```python
from build123d import *

# Parameters (mm, degrees)
SKETCH1_R                                    = 18.5
SKETCH1_R_2                                  = 2.125
MAIN_DEPTH                                   = 2
INLET_FILLET_R                               = 5
SKETCH20_R                                   = 8.5
FAN_PROTECTION_RIBS_DEPTH                    = 2
FAN_PROTECTION_RIBS_FILLETS_R                = 2
CSK_FOR_M4_HEX_SOCKET_COUNTERSUNK_HE_2_COUNT = 2
CSK_FOR_M4_HEX_SOCKET_COUNTERSUNK_HE_2_PITCH = 79.5
CSK_FOR_M4_HEX_SOCKET_COUNTERSUNK_HE_3_COUNT = 2
CSK_FOR_M4_HEX_SOCKET_COUNTERSUNK_HE_3_PITCH = 105.5
CSK_FOR_M4_HEX_SOCKET_COUNTERSUNK_HE_4_COUNT = 2
CSK_FOR_M4_HEX_SOCKET_COUNTERSUNK_HE_4_PITCH = 132.10034065


with BuildPart() as part:
    # Sketch1 → Main (new body)
    with BuildSketch(Plane.XY):
        with BuildLine():
            Line((-42.95, -46.393826455), (62.55, -46.393826455))
            ThreePointArc((62.55, -46.393826455), (67.782590181, -44.226416636), (69.95, -38.993826455))
            Line((69.95, -38.993826455), (69.95, 40.506173545))
            ThreePointArc((69.95, 40.506173545), (67.782590181, 45.738763726), (62.55, 47.906173545))
            Line((62.55, 47.906173545), (11.070508076, 47.906173545))
            Line((11.070508076, 47.906173545), (-23.570508076, 47.906173545))
            Line((-23.570508076, 47.906173545), (-42.95, 47.906173545))
            ThreePointArc((-42.95, 47.906173545), (-48.182590181, 45.738763726), (-50.35, 40.506173545))
            Line((-50.35, 40.506173545), (-50.35, -38.993826455))
            ThreePointArc((-50.35, -38.993826455), (-48.182590181, -44.226416636), (-42.95, -46.393826455))
        make_face()
        with Locations((-4.75, 17)):
            Circle(SKETCH1_R, mode=Mode.SUBTRACT)
        with Locations((-42.95, 40.506173545)):
            Circle(SKETCH1_R_2, mode=Mode.SUBTRACT)
        with Locations((-42.95, -38.993826455)):
            Circle(SKETCH1_R_2, mode=Mode.SUBTRACT)
        with Locations((62.55, 40.506173545)):
            Circle(SKETCH1_R_2, mode=Mode.SUBTRACT)
        with Locations((62.55, -38.993826455)):
            Circle(SKETCH1_R_2, mode=Mode.SUBTRACT)
    extrude(amount=-MAIN_DEPTH)

    # Inlet Fillet
    # the kernel refuses this fillet: 5 mm, written as the material it takes off along each edge
    with BuildSketch(Plane(origin=(-4.75, 17, 0), x_dir=(1, 0, 0), z_dir=(0, -1, 0))) as inlet_fillet_piece_1:
        with BuildLine():
            CenterArc((22.5, -5), INLET_FILLET_R, 90, 53.130102354)
            Line((22.5, 0), (22.5, 0.1))
            Line((22.5, 0.1), (18.5, 0.1))
            Line((18.5, 0.1), (18.4, 0))
            ThreePointArc((18.4, 0), (18.4, -1), (18.42, -1.94))
            Line((18.42, -1.94), (18.5, -2))
        make_face()
    revolve(axis=Axis((-4.75, 17, 0), (0, 0, 1)), mode=Mode.SUBTRACT)

    # Sketch20 → Fan Protection Ribs (add, through all)
    with BuildSketch(Plane.XY):
        with Locations((-4.75, 17)):
            Circle(SKETCH20_R)
        with BuildLine():
            ThreePointArc((-5.35, 25.478797084), (-4.75, 25.5), (-4.15, 25.478797084))
            Line((-4.15, 25.478797084), (-4.15, 39.491998577))
            ThreePointArc((-4.15, 39.491998577), (-4.75, 39.5), (-5.35, 39.491998577))
            Line((-5.35, 39.491998577), (-5.35, 25.478797084))
        make_face()
        with BuildLine():
            Line((15.02864215, 6.273615954), (2.892853669, 13.2802167))
            ThreePointArc((2.892853669, 13.2802167), (2.611215932, 12.75), (2.292853669, 12.240986215))
            Line((2.292853669, 12.240986215), (14.42864215, 5.234385469))
            ThreePointArc((14.42864215, 5.234385469), (14.735571585, 5.75), (15.02864215, 6.273615954))
        make_face()
        with BuildLine():
            ThreePointArc((-11.792853669, 12.240986215), (-12.111215932, 12.75), (-12.392853669, 13.2802167))
            Line((-12.392853669, 13.2802167), (-24.52864215, 6.273615954))
            ThreePointArc((-24.52864215, 6.273615954), (-24.235571585, 5.75), (-23.92864215, 5.234385469))
            Line((-23.92864215, 5.234385469), (-11.792853669, 12.240986215))
        make_face()
    extrude(amount=-FAN_PROTECTION_RIBS_DEPTH)

    # Fan Protection Ribs Fillets
    fan_protection_ribs_fillets_edges = [part.edges().sort_by_distance(p)[0] for p in [
        (-4.15, 25.478797084, -1),
        (2.892853669, 13.2802167, -1),
        (2.292853669, 12.240986215, -1),
        (-11.792853669, 12.240986215, -1),
        (-12.392853669, 13.2802167, -1),
        (-5.35, 25.478797084, -1),
    ]]
    fillet(fan_protection_ribs_fillets_edges, radius=FAN_PROTECTION_RIBS_FILLETS_R)

    # Sketch23 → CSK for M4 Hex Socket Countersunk Head Screw3 (revolve, cut)
    with BuildSketch(Plane(origin=(-42.95, 40.506173545, 0), x_dir=(0, -1, 0), z_dir=(1, 0, 0))):
        Polygon((0, 0), (0, 2), (2.15, 2), (2.15, 2.44), (4.59, 0), align=None)
    csk_for_m4_hex_socket_countersunk_head_s = revolve(axis=Axis((-42.95, 40.506173545, 6.35), (0, 0, -1)), mode=Mode.SUBTRACT)

    # CSK for M4 Hex Socket Countersunk He 2: CSK for M4 Hex Socket Countersunk Head Screw3 ×2
    with Locations(*[(0, -i * CSK_FOR_M4_HEX_SOCKET_COUNTERSUNK_HE_2_PITCH, 0) for i in range(1, CSK_FOR_M4_HEX_SOCKET_COUNTERSUNK_HE_2_COUNT)]):
        add(csk_for_m4_hex_socket_countersunk_head_s, mode=Mode.SUBTRACT)

    # CSK for M4 Hex Socket Countersunk He 3: CSK for M4 Hex Socket Countersunk Head Screw3 ×2
    with Locations(*[(i * CSK_FOR_M4_HEX_SOCKET_COUNTERSUNK_HE_3_PITCH, 0, 0) for i in range(1, CSK_FOR_M4_HEX_SOCKET_COUNTERSUNK_HE_3_COUNT)]):
        add(csk_for_m4_hex_socket_countersunk_head_s, mode=Mode.SUBTRACT)

    # CSK for M4 Hex Socket Countersunk He 4: CSK for M4 Hex Socket Countersunk Head Screw3 ×2
    with Locations(*[Vector(0.7986353364447739, -0.6018152535303031, 0) * (i * CSK_FOR_M4_HEX_SOCKET_COUNTERSUNK_HE_4_PITCH) for i in range(1, CSK_FOR_M4_HEX_SOCKET_COUNTERSUNK_HE_4_COUNT)]):
        add(csk_for_m4_hex_socket_countersunk_head_s, mode=Mode.SUBTRACT)


solid = part.part
```
Check sheet for the modelled part. Datum: model origin and axes. Units: mm. A direction names the side the tool comes from. Round coordinates to 2 decimals unless told otherwise and drop trailing zeros. One line per question, with ' | ' between items. Start each with the question number.
1. Release check for a two-part mould opening along X. For faces 1 (the face through (2.658, 21.168, -0.986)), 2 (the face through (9, -9, 0)), 3 (the face through (-48.12, 45.8, -0.99)) record: +X half, -X half, draft (parallel to the pull), parting line (faces both ways), or undercut.
2. Sectioned sample at A-A, the plane z = -0.75. Count the separate pieces of the cut face and the enclosed holes in it, then the cut area to 3 significant figures.
3. Scan lines: line 1 along Y through (x, z) = (10, -1.25); line 2 along X through (y, z) = (-40, -0.5); line 3 along Y through (x, z) = (-13.5, -1.5). Record each from-to range of solid material in increasing order. Write a range as from..to.
4. Set-up check for faces 4 (the face through (-17.484, 8.955, -0.986)), 5 (the face through (68, -44, -1)), 6 (the face through (-4.8, 8.5, -1)): record each of +Z, -Z, +X, -X, +Y, -Y from which the full face is reachable in a straight line by a thin tool's end or side.
Taken from the geometry:
1) face 1: undercut | face 2: draft | face 3: -X half
2) separate pieces: 1 | enclosed holes: 7 | area: 10,100 mm^2
3) line 1: y = -46.39..4.72, 7.79..9.18, 29.28..47.91 | line 2: x = -50.28..-46.91, -38.99..58.59, 66.51..69.88 | line 3: y = -46.39..0.21, 11.26..12.7, 33.79..47.91
4) face 4: +Z | face 5: +Z, -Z, +X, -Y | face 6: +Z, -Z
